```python
from build123d import *

# Parameters (mm, degrees)
BOSS_EXTRU_1_DEPTH      = 5
ESQUISSE3_R             = 2.75
BOSS_EXTRU_2_DEPTH      = 5
ESQUISSE4_R             = 3.25
BOSS_EXTRU_3_DEPTH      = 4
ESQUISSE5_W             = 10
ESQUISSE5_H             = 2
ENL_V_MAT_EXTRU_1_DEPTH = 9


with BuildPart() as part:
    # Esquisse1 → Boss.-Extru.1 (new body)
    with BuildSketch(Plane.XY):
        with BuildLine():
            Line((-111.881065478, -43.864420881), (-124.856118958, 10.611702211))
            ThreePointArc((-124.856118958, 10.611702211), (-119.297939992, 19.645341931), (-110.264300273, 14.087162965))
            Line((-110.264300273, 14.087162965), (-97.289246792, -40.388960128))
            ThreePointArc((-97.289246792, -40.388960128), (-102.847425758, -49.422599847), (-111.881065478, -43.864420881))
        make_face()
    extrude(amount=BOSS_EXTRU_1_DEPTH)

    # Esquisse3 → Boss.-Extru.2 (add)
    with BuildSketch(Plane.XY):
        with Locations((-117.560209615, 12.349432588)):
            Circle(ESQUISSE3_R)
        with Locations((-104.585156135, -42.126690504)):
            Circle(ESQUISSE3_R)
    extrude(amount=-BOSS_EXTRU_2_DEPTH)

    # Esquisse4 → Boss.-Extru.3 (add)
    with BuildSketch(Plane(origin=(0, 0, -5), x_dir=(-1, 0, 0), z_dir=(0, 0, -1))):
        with Locations((117.560209615, 12.349432588)):
            Circle(ESQUISSE4_R)
        with Locations((104.585156135, -42.126690504)):
            Circle(ESQUISSE4_R)
    extrude(amount=BOSS_EXTRU_3_DEPTH)

    # Esquisse5 → Enlèv. mat.-Extru.1 (cut)
    with BuildSketch(Plane(origin=(0, 0, -9), x_dir=(-1, 0, 0), z_dir=(0, 0, -1))):
        with Locations((104.585156135, -42.126690504)):
            Rectangle(ESQUISSE5_W, ESQUISSE5_H)
        with Locations((117.560209615, 12.349432588)):
            Rectangle(ESQUISSE5_W, ESQUISSE5_H)
    extrude(amount=-ENL_V_MAT_EXTRU_1_DEPTH, mode=Mode.SUBTRACT)


solid = part.part
```
Can you work these out from the model? Positions are in its coordinate system, mm. A direction names the side the tool comes from. Round coordinates to 2 decimals unless told otherwise and drop trailing zeros. Loops run counter-clockwise (first coordinate to the right, second up) from the corner with the lowest first, then second, coordinate; pieces in that order, holes last. Notation, with made-up numbers: (74, 56.5) -> (104, 56.5) arc R21 cw to (104, 84.5) -> close; hole circle Ø2 at (48, -29.5). An arc over 180 degrees is marked (long way). Answer in a Markdown table with one row per item.
Item 1: We'd pull the mould along Y, two halves only. Please class faces 1 (the cylindrical face through (-117.5, 9.1, -7)), 2 (the flat face through (-105, -44, -9)), 3 (the flat face through (-118, 11.349, -5)): released by +Y, released by -Y, zero draft, split by the parting line, or undercut.
Answer block:
| item | result |
|---|---|
| face 1 | released by -Y |
| face 2 | zero draft |
| face 3 | undercut |
Item 2: Suppose I cut it at C-C, the plane z = -5.75. List the corners of the cut face in (x, y) for me.
Answer block:
| item | result |
|---|---|
| outline | (-120.65, 11.35) arc R3.25 ccw to (-114.47, 11.35) -> close; (-120.65, 13.35) -> (-114.47, 13.35) arc R3.25 ccw to start; (-107.68, -43.13) arc R3.25 ccw to (-101.49, -43.13) -> close; (-107.68, -41.13) -> (-101.49, -41.13) arc R3.25 ccw to start |
Item 3: On a 3-axis mill with a long thin cutter (end or side, diameter ignored), from which of +Z, -Z, +X, -X, +Y, -Y can I reach the whole of each face in a straight line? I mean faces 4 (the flat face through (-104.6, -39.2, -5)), 5 (the cylindrical face through (-117.6, 15.6, -7)), 6 (the flat face through (-105, -45, -5)). Say none if no direction works.
Answer block:
| item | result |
|---|---|
| face 4 | +Y |
| face 5 | -Z, +Y |
| face 6 | -Y |
Item 4: If I drill on probe 1 along Y at (x, z) = (-117.5, -5.5); probe 2 along Y at (x, z) = (-117.5, -0.25); probe 3 along Z at (x, y) = (-105.25, -35), over which ranges is the centre line in solid material (lowest first)?
Answer block:
| item | result |
|---|---|
| probe 1 | 9.1 to 11.35, 13.35 to 15.6 |
| probe 2 | 9.6 to 11.35, 13.35 to 15.1 |
| probe 3 | 0 to 5 |
Item 5: Suppose I cut it at D-D, the plane z = 3.5. List the corners of the cut face in (x, y) for me.
Answer block:
| item | result |
|---|---|
| outline | (-124.86, 10.61) -> (-111.88, -43.86) arc R7.5 ccw to (-97.29, -40.39) -> (-110.26, 14.09) arc R7.5 ccw to start |
Item 6: Suppose I cut it at B-B, the plane x = -103.75. List the corners of the cut face in (y, z) for me.
Answer block:
| item | result |
|---|---|
| outline | (-49.58, 0) -> (-44.75, 0) -> (-44.75, -5) -> (-45.27, -5) -> (-45.27, -9) -> (-43.13, -9) -> (-43.13, 0) -> (-41.13, 0) -> (-41.13, -9) -> (-38.99, -9) -> (-38.99, -5) -> (-39.51, -5) -> (-39.51, 0) -> (-13.26, 0) -> (-13.26, 5) -> (-49.58, 5) -> close |
Item 7: Suppose I cut it at A-A, the plane z = -2.5. List the corners of the cut face in (x, y) for me.
Answer block:
| item | result |
|---|---|
| outline | (-120.12, 11.35) arc R2.75 ccw to (-115, 11.35) -> close; (-120.12, 13.35) -> (-115, 13.35) arc R2.75 ccw to start; (-107.15, -43.13) arc R2.75 ccw to (-102.02, -43.13) -> close; (-107.15, -41.13) -> (-102.02, -41.13) arc R2.75 ccw to start |
Item 8: Will these pins go through, and if not, where does the flat tip stop? P1, Ø1.9, axis at x = -116, z = -5, coming from the +Y side; P2, Ø3, axis at x = -118.5, z = -6, coming from the +Y side; P3, Ø4, axis at x = -112, y = -5.5, coming from the -Z side.
Answer block:
| item | result |
|---|---|
| P1 | y = 15.54 |
| P2 | y = 15.6 |
| P3 | z = 0 |
